The drawing under review shows one solid part. Ordinate dimensions are in mm from its lowest x, y, z. A direction names the side the tool comes from. Coordinates: 2 decimals unless noted, no trailing zeros. Order: outer loops, then holes, each group sorted by start corner. A loop starts at its lowest first (then second) coordinate and runs counter-clockwise, first axis right, second up.
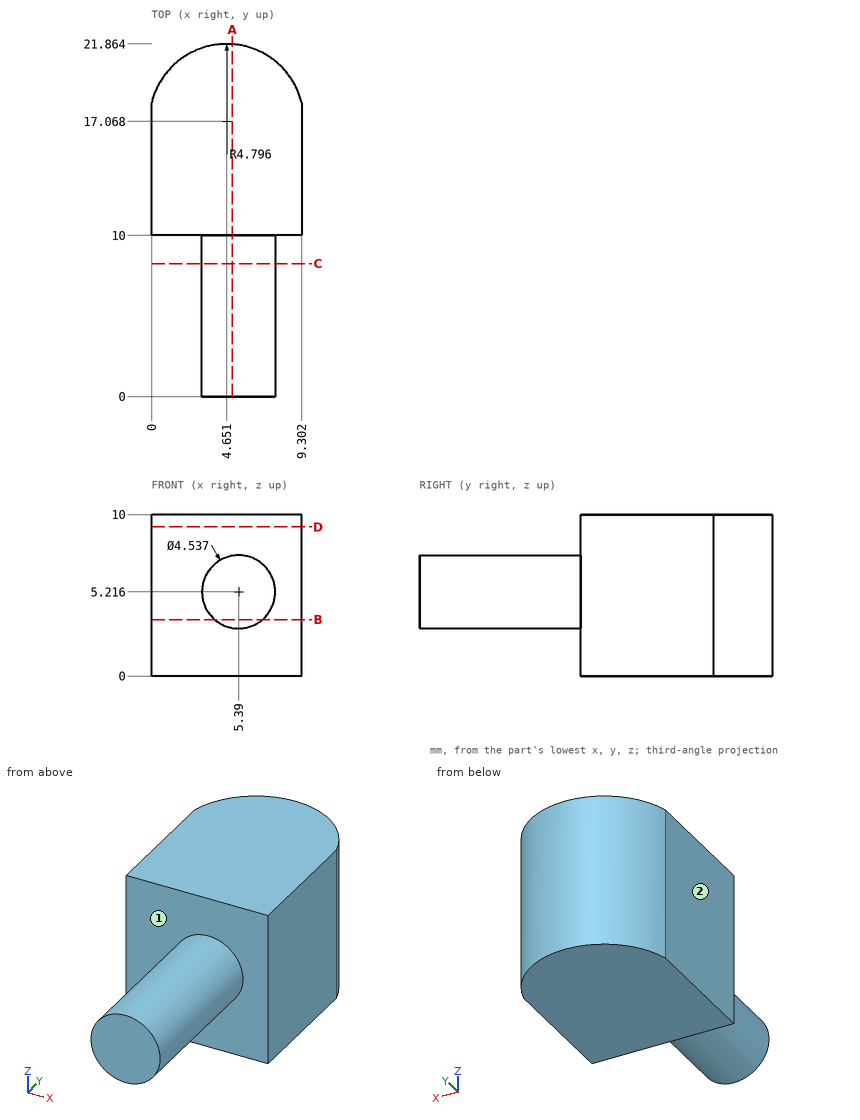
1. Take a section at B-B, the plane z = 3.5. Give the boundary of the cut face in (x, y) (1 decimal).
Answer below:
outline: (0, 10) - (3.9, 10) - (3.9, 0) - (6.9, 0) - (6.9, 10) - (9.3, 10) - (9.3, 18.2) arc R4.8 ccw to (0, 18.2) - close
2. To check wall thickness, follow L1, parallel to Y at x = 4.75, z = 1.5; L2, parallel to Y at x = 1.5, z = 6.25 (1 decimal); L3, parallel to X at y = 18.25, z = 2. State the ranges of each line that lie inside material, in increasing order.
Answer below:
L1: y = 10 to 21.86
L2: y = 10 to 20.7
L3: x = 0 to 9.3
3. Take a section at A-A, the plane x = 5. Give the boundary of the cut face in (y, z).
Answer below:
outline: (0, 2.98) - (10, 2.98) - (10, 0) - (21.85, 0) - (21.85, 10) - (10, 10) - (10, 7.45) - (0, 7.45) - close
4. Take a section at C-C, the plane y = 8.25. Give the boundary of the cut face in (x, z) (1 decimal), plus the area to 3 significant figures.
Answer below:
outline: circle Ø4.5 at (5.4, 5.2)
area: 16.2 mm2
5. Machinability: for the marked faces 1 and 2, which of the approach directions +Z, -Z, +X, -X, +Y, -Y give a long, thin tool a straight path to every point of the face, cutting with its end or side? Answer none if there is none.
Answer below:
face 1: -Y
face 2: +Z, -Z, -X, +Y, -Y
6. Take a section at D-D, the plane z = 9.25. Give the boundary of the cut face in (x, y) (1 decimal).
Answer below:
outline: (0, 10) - (9.3, 10) - (9.3, 18.2) arc R4.8 ccw to (0, 18.2) - close
